The listing builds one solid part. Answer for the finished solid, in the listing's coordinates (mm). A direction names the side the tool comes from. Give positions to 0.01 mm unless a question says otherwise; leave off trailing zeros. Write each loop counter-clockwise with the first axis right and the second up, starting at its lowest first coordinate (ties: lowest second). Pieces come first, ordered by that corner, then holes. Notation, with made-up numbers: M -37.5,33 L -4.5,33 A24 ccw -4.5,46 Z; hole C -36,88 d2. An arc over 180 degrees is marked long. Answer as a JSON object with one key per item and string values.
```python
from build123d import *

# Parameters (mm, degrees)
CROQUIS5_R                   = 5
SALIENTE_EXTRUIR2_DEPTH      = 70
CROQUIS6_R                   = 4
SALIENTE_EXTRUIR3_DEPTH      = 50
CROQUIS7_R                   = 5
SALIENTE_EXTRUIR4_DEPTH      = 30
SALIENTE_EXTRUIR5_DEPTH      = 5
SALIENTE_EXTRUIR5_DEPTH_BACK = 20
CROQUIS8_R                   = 4
CROQUIS10_W                  = 10
CROQUIS10_H                  = 30
SALIENTE_EXTRUIR6_DEPTH      = 30
CROQUIS11_W                  = 60
CROQUIS11_H                  = 170
SALIENTE_EXTRUIR7_DEPTH      = 70


with BuildPart() as part:
    # Croquis5 → Saliente-Extruir2 (new body)
    with BuildSketch(Plane(origin=(0, 0, 0), x_dir=(1, 0, 0), z_dir=(0, 1, 0))):
        with Locations(Location((0, 0, 0), (0, 0, 270))):
            Circle(CROQUIS5_R)
    extrude(amount=SALIENTE_EXTRUIR2_DEPTH)

    # Croquis6 → Saliente-Extruir3 (add)
    with BuildSketch(Plane.XY):
        with Locations(Location((0, 6, 0), (0, 0, 180))):
            Circle(CROQUIS6_R)
    extrude(amount=SALIENTE_EXTRUIR3_DEPTH)

    # Croquis7 → Saliente-Extruir4 (add)
    with BuildSketch(Plane.XY.offset(50)):
        with Locations((0, 6)):
            Circle(CROQUIS7_R)
    extrude(amount=SALIENTE_EXTRUIR4_DEPTH)

    # Croquis8 → Saliente-Extruir5 (add, two sides: drawn at the far end of the back side and taken through both)
    with BuildSketch(Plane(origin=(0, 0, 0), x_dir=(1, 0, 0), z_dir=(0, 1, 0)).offset(-SALIENTE_EXTRUIR5_DEPTH_BACK)):
        with Locations(Location((0, -74, 0), (0, 0, 90))):
            Circle(CROQUIS8_R)
    extrude(amount=SALIENTE_EXTRUIR5_DEPTH + SALIENTE_EXTRUIR5_DEPTH_BACK)

    # Croquis10 → Saliente-Extruir6 (add)
    with BuildSketch(Plane.XZ.offset(20)):
        with Locations((0, 74)):
            Rectangle(CROQUIS10_W, CROQUIS10_H)
    extrude(amount=SALIENTE_EXTRUIR6_DEPTH)

    # Croquis11 → Saliente-Extruir7 (add)
    with BuildSketch(Plane(origin=(0, 70, 0), x_dir=(1, 0, 0), z_dir=(0, 1, 0))):
        with Locations((-10, -70)):
            Rectangle(CROQUIS11_W, CROQUIS11_H)
    extrude(amount=SALIENTE_EXTRUIR7_DEPTH)


solid = part.part
```
1. For faces 5 (the flat face through (0, 0, 0)), 6 (the flat face through (0, -35, 89)), 7 (the flat face through (5, -35, 74)), 8 (the cylindrical face through (0, -9, 78)), determine the directions among +Z, -Z, +X, -X, +Y, -Y from which every point of the face is accessible in a straight line to the end or side of a thin tool.
Verdict:
{"face 5": "-Z, +X, -X, -Y", "face 6": "+Z, +X, -X, -Y", "face 7": "+Z, -Z, +X, -Y", "face 8": "none"}
2. The mould has two halves that part along Z. Classify faces 1 (the flat face through (0, 6, 80)), 2 (the flat face through (2, -20, 78)), 3 (the flat face through (-10, 105, -15)), 4 (the cylindrical face through (0.867, 9.905, 26.171)): released by +Z, released by -Z, zero draft, split by the parting line, or undercut.
Verdict:
{"face 1": "released by +Z", "face 2": "zero draft", "face 3": "released by -Z", "face 4": "undercut"}
3. A cutting plane is placed at D-D, the plane y = 6. Give the vertices of the cut face in (x, z), plus the area to 3 significant figures.
Verdict:
{"outline": "M -5,50 L -4,50 L -4,3 A5 ccw long 4,3 L 4,50 L 5,50 L 5,80 L -5,80 Z", "area": "743 mm2"}
4. Flat-ended cylindrical pins translate along their axes: pin 1 (11 mm diameter, centred on x = 1.5, z = -1, fed in from -Y); pin 2 (2 mm diameter, centred on x = 3.5, z = 91, fed in from -Y); pin 3 (24 mm diameter, centred on y = -36.5, z = 70, fed in from +X). Find the tip coordinate at first contact, or state that the pin passes through.
Verdict:
{"pin 1": "stops at y = 0", "pin 2": "stops at y = 70", "pin 3": "stops at x = 5"}
5. Consider line 1 along Y through (x, z) = (-1.5, 88.5); line 2 along X through (y, z) = (5.5, 23); line 3 along Y through (x, z) = (-4, 94.5). Determine where each line is inside the solid, lowest interval first.
Verdict:
{"line 1": "y = -50 to -20, 70 to 140", "line 2": "x = -3.97 to 3.97", "line 3": "y = 70 to 140"}
6. A cutting plane is placed at B-B, the plane z = 0. Give the vertices of the cut face in (x, y).
Verdict:
{"outline": "M -40,70 L -5,70 L -5,0 L 5,0 L 5,70 L 20,70 L 20,140 L -40,140 Z"}
7. A cutting plane is placed at C-C, the plane z = 33. Give the vertices of the cut face in (x, y).
Verdict:
{"outline": "M -40,70 L 20,70 L 20,140 L -40,140 Z; C 0,6 d8"}
8. A cutting plane is placed at A-A, the plane x = 0. Give the vertices of the cut face in (y, z), plus the area to 3 significant figures.
Verdict:
{"outline": "M -50,59 L -20,59 L -20,70 L 1,70 L 1,50 L 2,50 L 2,5 L 0,5 L 0,-5 L 70,-5 L 70,-15 L 140,-15 L 140,155 L 70,155 L 70,5 L 10,5 L 10,50 L 11,50 L 11,80 L 1,80 L 1,78 L -20,78 L -20,89 L -50,89 Z", "area": "14,300 mm2"}
